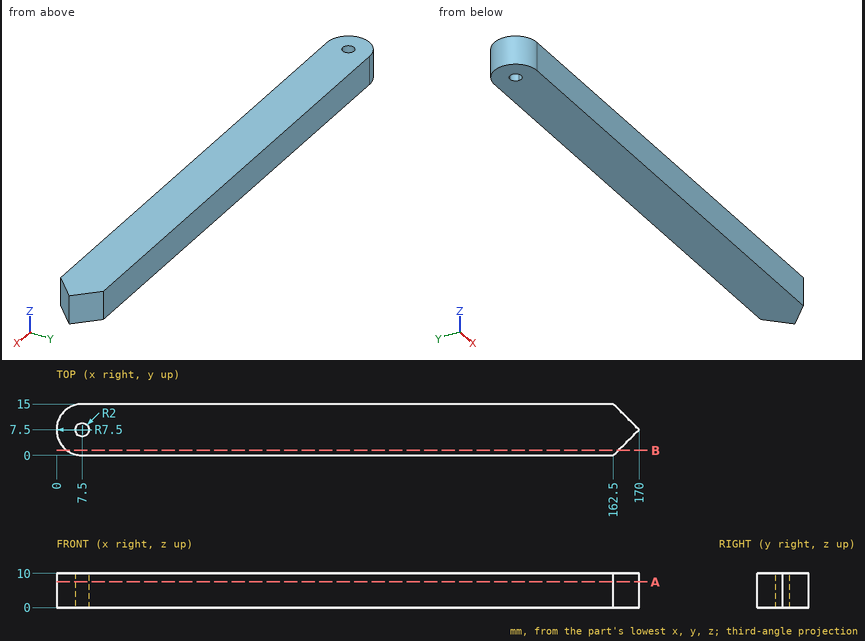
For this review, use the dimensioned drawing (mm, ordinates from the lowest corner) and the shaded views. Coordinates: 2 decimals unless noted, no trailing zeros. Write each loop counter-clockwise with the first axis right and the second up, starting at its lowest first coordinate (ties: lowest second). Pieces come first, ordered by that corner, then holes. Notation, with made-up numbers: (48, -4.5) -> (58, -4.5) arc R16 cw to (58, 26.5) -> close; hole circle Ø3 at (-8, 82). An arc over 180 degrees is marked (long way). Write each question's results on one line, items separated by ' | '. Start each with the question number.
(1) Take a section at B-B on y = 1.5. Write out the cut boundary in (x, z), and give its area (3 significant figures).
(2) For line 1 along X through (y, z) = (7.25, 7); line 2 along X through (y, z) = (6.25, 7.25); line 3 along X through (y, z) = (5.25, 4.5), list the stretches that pass through material, from the lowest coordinate up. Write a range as from..to.
(3) Take a section at A-A on z = 7.5. Write out the cut boundary in (x, y).
(4) Clearance check with flat-ended pins moving along their axes: P1, Ø6, axis at x = 101, y = 5, coming from the -Z side; P2, Ø3, axis at y = 6.5, z = 5.5, coming from the +X side; P3, Ø5, axis at y = 2, z = 1, coming from the +X side. State where each tip first meets the part, or that it passes through.
Results found:
1) outline: (3, 0) -> (164, 0) -> (164, 10) -> (3, 10) -> close | area: 1,610 mm2
2) line 1: x = 0..5.52, 9.48..169.75 | line 2: x = 0.1..5.94, 9.06..168.75 | line 3: x = 0.35..167.75
3) outline: (7.5, 0) -> (162.5, 0) -> (170, 7.5) -> (162.5, 15) -> (7.5, 15) arc R7.5 ccw to start; hole (7.5, 5.5) arc R2 ccw to (9.5, 7.5) arc R2 ccw to (7.5, 9.5) arc R2 ccw to start
4) P1: stops at z = 0 | P2: stops at x = 170 | P3: stops at x = 167
